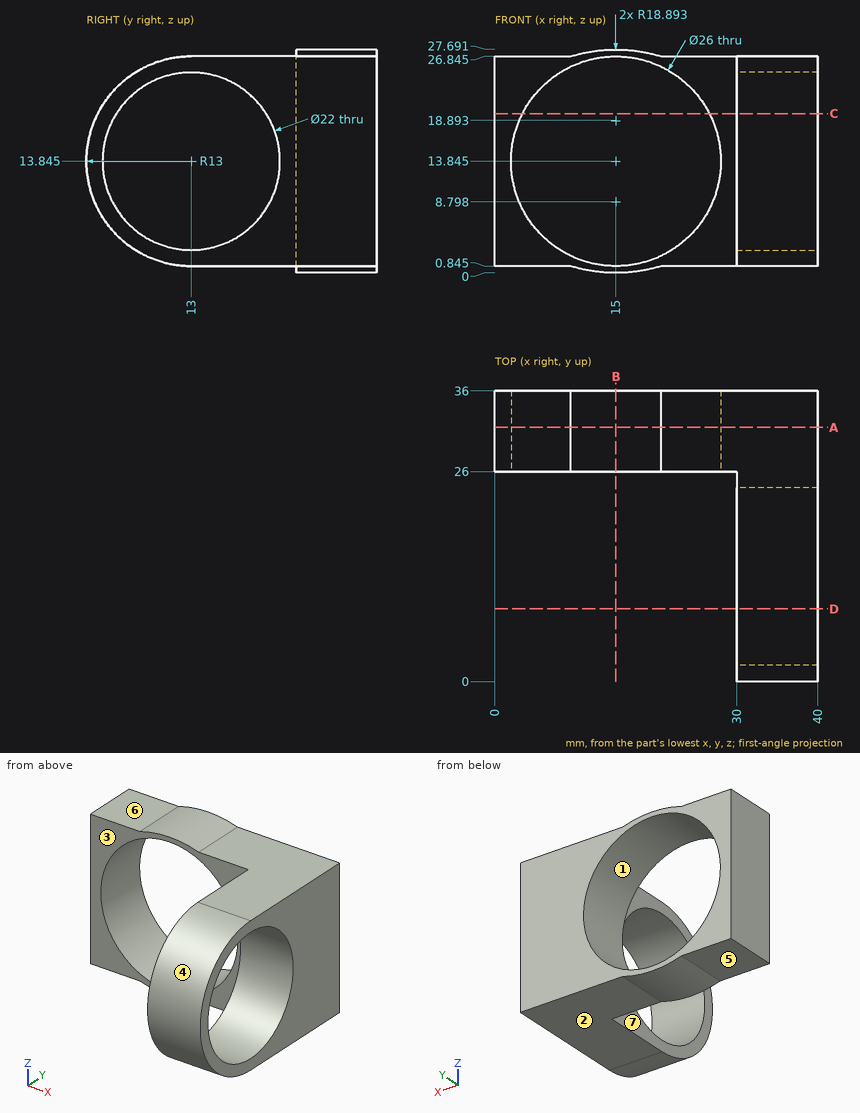
Answer from the drawing. Dimensions are ordinates in mm from the lowest x, y and z of the part. A direction names the side the tool comes from. Round coordinates to 2 decimals unless told otherwise and drop trailing zeros. Loops run counter-clockwise (first coordinate to the right, second up) from the corner with the lowest first, then second, coordinate; pieces in that order, holes last.
Q1. Consider probe 1 along Y at (x, z) = (10.5, 26.75); probe 2 along Y at (x, z) = (30.5, 13); probe 3 along Z at (x, y) = (37.5, 12). Determine where each line is inside the solid, lowest interval first.
Q2. Each of these flat-tipped pins is pushed along its axis until it touches: pin 1 (8.5 mm diameter, centred on x = 10, z = 18.5, fed in from -Y); pin 2 (15.5 mm diameter, centred on x = 31, y = 26.5, fed in from +Z) (1 decimal); pin 3 (3 mm diameter, centred on x = 31.5, z = 17, fed in from -Y); pin 4 (15.5 mm diameter, centred on x = 30.5, y = 21.5, fed in from -Z) (1 decimal). Where does it stop, or does it pass through?
Q3. Section C-C on z = 19.75 is taken. Write down the section's boundary in (x, y).
Q4. Which of the six approach directions +Z, -Z, +X, -X, +Y, -Y give full straight-line access (tool end or side, diameter ignored) to the marked faces 5, 6 and 7?
Q5. Section B-B on x = 15 is taken. Write down the section's boundary in (y, z) (1 decimal), and give its area (3 significant figures).
Q6. Section D-D on y = 9 is taken. Write down the section's boundary in (x, z) (1 decimal).
Q7. Determine the mould class of the marked faces 1, 2, 3 and 4 for opening direction Z: released by +Z, released by -Z, zero draft, split by the parting line, or undercut.
Q8. Section A-A on y = 31.5 is taken. Write down the section's boundary in (x, z) (1 decimal).
Output:
1. probe 1: y = 26 to 36
1. probe 2: y = 0.03 to 2.03, 23.97 to 36
1. probe 3: z = 0.88 to 2.89, 24.8 to 26.81
2. pin 1: passes through
2. pin 2: stops at z = 26.8
2. pin 3: stops at y = 0.11
2. pin 4: stops at z = 0.8
3. outline: (0, 26) - (3.42, 26) - (3.42, 36) - (0, 36) - close; (26.58, 26) - (30, 26) - (30, 22.28) - (40, 22.28) - (40, 36) - (26.58, 36) - close; (30, 1.42) - (40, 1.42) - (40, 3.72) - (30, 3.72) - close
4. face 5: -Z, -X, +Y, -Y
4. face 6: +Z, -X, +Y, -Y
4. face 7: +Z, -Z, -X, -Y
5. outline: (26, 0) - (36, 0) - (36, 0.8) - (26, 0.8) - close; (26, 26.8) - (36, 26.8) - (36, 27.7) - (26, 27.7) - close
5. area: 16.9 mm2
6. outline: (30, 1.5) - (40, 1.5) - (40, 3.6) - (30, 3.6) - close; (30, 24.1) - (40, 24.1) - (40, 26.2) - (30, 26.2) - close
7. face 1: undercut
7. face 2: released by -Z
7. face 3: zero draft
7. face 4: split by the parting line
8. outline: (0, 0.8) - (9.4, 0.8) arc R18.9 ccw to (20.6, 0.8) - (40, 0.8) - (40, 26.8) - (20.6, 26.8) arc R18.9 ccw to (9.4, 26.8) - (0, 26.8) - close; hole circle Ø26 at (15, 13.8)
